Input: part model. Units: mm. Frame: model coordinates. A direction names the side the tool comes from. Coordinates: 2 decimals unless noted, no trailing zeros. Order: outer loops, then holes, each group sorted by start corner. A loop starts at its lowest first (then second) coordinate and runs counter-clockwise, first axis right, second up. Notation, with made-up numbers: (89, 2.25) - (145, 2.25) arc R22 ccw to (145, 32.25) - close; hole circle Ø7 at (47, -22). An arc over 180 degrees is marked (long way). Use a Markdown table: item, result. Add a question column.
from build123d import *

# Parameters (mm, degrees)
BOSS_EXTRUDE1_DEPTH = 4


with BuildPart() as part:
    # Sketch1 → Boss-Extrude1 (new, symmetric)
    with BuildSketch(Plane(origin=(0, 0, 0), x_dir=(1, 0, 0), z_dir=(0, 1, 0))):
        with BuildLine():
            Line((-20, 0), (0, 0))
            Line((0, 0), (20, 0))
            Line((20, 0), (20, -2.8))
            Line((20, -2.8), (24, -2.8))
            Line((24, -2.8), (24, -14.220649169))
            ThreePointArc((24, -14.220649169), (0, -13.5), (-24, -14.220649169))
            Line((-24, -14.220649169), (-24, -2.8))
            Line((-24, -2.8), (-20, -2.8))
            Line((-20, -2.8), (-20, 0))
        make_face()
    extrude(amount=BOSS_EXTRUDE1_DEPTH, both=True)


solid = part.part
1) Cut plane A-A (y = 2). Return the cut outline in (x, z), and give its area (3 significant figures).
2) Reachability of faces 5 (the flat face through (-22, 0, 2.8)), 6 (the flat face through (24, 0, 8)) from +Z, -Z, +X, -X, +Y, -Y: full face, straight path, thin tool, end or side. Return the list, or none.
3) Cut plane B-B (x = 18.5). Return the cut outline in (y, z).
4) Contact query for flat-ended pins moving along their axis: P1, Ø2, axis at x = 22.5, y = 1, coming from the -Z side; P2, Ø2, axis at y = 1, z = 1, coming from the -X side; P3, Ø3, axis at x = -12, y = -3, coming from the +Z side. Output: stop coordinate, or through.
5) Pull-direction query (X, two-part tool) for faces 1 (the flat face through (20, 0, 1)), 2 (the flat face through (22, 0, 2.8)), 3 (the cylindrical face through (0.3, 0.1, 13.5)), 4 (the flat face through (-24, 0, 9)); classes: pulls with the +X half, pulls with the -X half, needs draft (parallel to the pull), parting line crosses it, or undercut.
6) Cut plane C-C (x = -3). Return the cut outline in (y, z), and give its area (3 significant figures).
7) Material intervals for L1, parallel to X at y = 1, z = 2.5; L2, parallel to Z at x = 0, y = 0; L3, parallel to Z at x = -8, y = 2.5, sorted ascending.
Computed:
| question | item | result |
|---|---|---|
| 1 | outline | (-24, 2.8) - (-20, 2.8) - (-20, 0) - (20, 0) - (20, 2.8) - (24, 2.8) - (24, 14.22) arc R400 cw to (-24, 14.22) - close |
| 1 | area | 637 mm2 |
| 2 | face 5 | -Z, -X, +Y, -Y |
| 2 | face 6 | +Z, -Z, +X, +Y, -Y |
| 3 | outline | (-4, 0) - (4, 0) - (4, 13.93) - (-4, 13.93) - close |
| 4 | P1 | stops at z = 2.8 |
| 4 | P2 | stops at x = -20 |
| 4 | P3 | stops at z = 13.73 |
| 5 | face 1 | pulls with the +X half |
| 5 | face 2 | needs draft |
| 5 | face 3 | undercut |
| 5 | face 4 | pulls with the -X half |
| 6 | outline | (-4, 0) - (4, 0) - (4, 13.51) - (-4, 13.51) - close |
| 6 | area | 108 mm2 |
| 7 | L1 | x = -20 to 20 |
| 7 | L2 | z = 0 to 13.5 |
| 7 | L3 | z = 0 to 13.58 |
